Verification items for the finished model (mm, model axes). A direction names the side the tool comes from. Give positions to 0.01 mm unless a question says otherwise; leave off trailing zeros. Order: outer loops, then holes, each group sorted by start corner. A loop starts at its lowest first (then second) coordinate and runs counter-clockwise, first axis right, second up.
(1) Sectioned sample at A-A on z = -67.5. Record the cut outline in (x, y), plus the area to 3 significant figures.
(2) Gauge pin test, flat ends, axial feed: pin 1 (8 mm diameter, centred on x = 87, z = -36, fed in from -Y); pin 2 (3 mm diameter, centred on x = 90.5, z = 69, fed in from +Y). Record the tip position at first contact, or that the pin passes through.
(3) Access from +Z, -Z, +X, -X, +Y, -Y to the whole of each face (thin tool, end or side, straight path). Record for faces 1 (the face through (-84, 2, -32)), 2 (the face through (2, 2, -75)), 3 (the face through (-85.12, 3.99, 66.42)).
(4) Scan lines: L1, parallel to X at y = 0.9, z = -36; L2, parallel to X at y = 4.7, z = -36; L3, parallel to Z at x = -87, y = 2.4. Record each from-to range of solid material in increasing order.
(5) Mould release check, pull along X, two halves, no side actions. Record for faces 4 (the face through (-85.12, 3.99, -68.58)), 5 (the face through (84.52, 4.51, 36.33)), 6 (the face through (120, 2, 1)), 7 (the face through (-2, 2, 75)): pulls with the +X half, pulls with the -X half, needs draft (parallel to the pull), parting line crosses it, or undercut.
Autodesk Inventor part; units mm, degrees
ref_plane "YZ Plane" through (0, 0, 0) normal (1, 0, 0) x (0, 1, 0)
ref_plane "XZ Plane" through (0, 0, 0) normal (0, 1, 0) x (-1, 0, 0)
ref_plane "XY Plane" through (0, 0, 0) normal (0, 0, 1) x (1, 0, 0)
sketch "Sketch1" plane through (0, 0, 0) normal (0, 1, 0) x (-1, 0, 0)
  line L0 (-120, -75) -> (120, -75)
  line L1 (120, -75) -> (120, 75)
  line L2 (120, 75) -> (-120, 75)
  line L3 (-120, 75) -> (-120, -75)
  line L4 (-120, -75) -> (120, 75) construction
  line L5 (120, -75) -> (-120, 75) construction
  point P0 (0, 0)
  dimension "d0" = 240
  dimension "d1" = 150
extrude "Extrusion1" add sketch "Sketch1" along normal blind 5
sketch "Sketch2" plane through (0, 0, 0) normal (0, 1, 0) x (1, 0, 0)
  line L0 (-120, 75) -> (-120, -75)
  line L1 (-120, -75) -> (120, -75)
  line L2 (120, -75) -> (120, 75)
  line L3 (120, 75) -> (-120, 75)
  line L4 (-87, -36) -> (87, -36) construction
  line L5 (87, -36) -> (87, 36) construction
  line L6 (87, 36) -> (-87, 36) construction
  line L7 (-87, 36) -> (-87, -36) construction
  line L8 (-120, 0) -> (-87, 0) construction
  line L9 (0, 36) -> (0, 75) construction
  line L10 (0, -36) -> (0, -75) construction
  line L11 (87, 0) -> (120, 0) construction
  point P0 (0, 0)
  dimension "d4" = 72
  dimension "d5" = 174
hole "Hole1" at (-87, 0, 36) at (-87, 0, -36) at (87, 0, -36) at (87, 0, 36) direction (0, 1, 0) diameter 5 end through all counterbore diameter 10 counterbore depth 4
sketch "Sketch3" plane through (0, 5, 0) normal (0, 1, 0) x (1, 0, 0)
  line L0 (-90, -67.5) -> (90, -67.5) construction
  line L1 (90, -67.5) -> (90, 67.5) construction
  line L2 (90, 67.5) -> (-90, 67.5) construction
  line L3 (-90, 67.5) -> (-90, -67.5) construction
  line L4 (-90, -67.5) -> (90, 67.5) construction
  line L5 (90, -67.5) -> (-90, 67.5) construction
  point P0 (0, 0)
  dimension "d13" = 180
  dimension "d14" = 135
hole "Hole2" at (90, 5, -67.5) at (90, 5, 67.5) at (-90, 5, 67.5) at (-90, 5, -67.5) direction (0, -1, 0) diameter 5 end through all counterbore diameter 10 counterbore depth 2
properties part number "Hotplate Mount"
Ans:
1. outline: (-120, 0) - (-92.5, 0) - (-92.5, 3) - (-95, 3) - (-95, 5) - (-120, 5) - close; (-87.5, 0) - (87.5, 0) - (87.5, 3) - (85, 3) - (85, 5) - (-85, 5) - (-85, 3) - (-87.5, 3) - close; (92.5, 0) - (120, 0) - (120, 5) - (95, 5) - (95, 3) - (92.5, 3) - close
1. area: 1,130 mm2
2. pin 1: stops at y = 4
2. pin 2: stops at y = 3
3. face 1: -Y
3. face 2: -Z, +X, -X, +Y, -Y
3. face 3: +Y
4. L1: x = -120 to -92, -82 to 82, 92 to 120
4. L2: x = -120 to -89.5, -84.5 to 84.5, 89.5 to 120
4. L3: z = -75 to -41, -31 to 31, 41 to 75
5. face 4: undercut
5. face 5: undercut
5. face 6: pulls with the +X half
5. face 7: needs draft
